from build123d import *

# Parameters (mm, degrees)
SKETCH1_R           = 2.075
SKETCH1_R_2         = 5
BOSS_EXTRUDE1_DEPTH = 5
BOSS_EXTRUDE2_DEPTH = 10


with BuildPart() as part:
    # Sketch1 → Boss-Extrude1 (new body)
    with BuildSketch(Plane(origin=(0, 0, 0), x_dir=(1, 0, 0), z_dir=(0, 1, 0))):
        with BuildLine():
            ThreePointArc((23, 37.81190645), (-17.889435034, 76.754473357), (16.937219731, 121.201897721))
            Line((16.937219731, 121.201897721), (16.937219731, 130.106631122))
            ThreePointArc((16.937219731, 130.106631122), (-26.790527996, 80.780951543), (15, 29.80360013))
            Line((15, 29.80360013), (15, 17.435595774))
            ThreePointArc((15, 17.435595774), (-20.90454496, -9.591663047), (23, 0))
            Line((23, 0), (23, 37.81190645))
        make_face()
        with Locations(Location((8, 8, 0), (0, 0, 270))):
            Circle(SKETCH1_R, mode=Mode.SUBTRACT)
        with Locations(Location((0, 0, 0), (0, 0, 270))):
            Circle(SKETCH1_R_2, mode=Mode.SUBTRACT)
        with Locations(Location((-8, -8, 0), (0, 0, 270))):
            Circle(SKETCH1_R, mode=Mode.SUBTRACT)
        with Locations(Location((-8, 8, 0), (0, 0, 270))):
            Circle(SKETCH1_R, mode=Mode.SUBTRACT)
        with Locations(Location((8, -8, 0), (0, 0, 270))):
            Circle(SKETCH1_R, mode=Mode.SUBTRACT)
    extrude(amount=BOSS_EXTRUDE1_DEPTH)

    # Sketch1_3 → Boss-Extrude2 (add)
    with BuildSketch(Plane(origin=(0, 0, 0), x_dir=(1, 0, 0), z_dir=(0, 1, 0))):
        with BuildLine():
            Line((23, 23), (23, 29))
            Line((23, 29), (23, 29.009843473))
            Line((23, 29.009843473), (23, 37.81190645))
            ThreePointArc((23, 37.81190645), (19.957969223, 37.994952611), (16.937219731, 38.398102279))
            ThreePointArc((16.937219731, 38.398102279), (-18, 79.8), (16.937219731, 121.201897721))
            Line((16.937219731, 121.201897721), (16.937219731, 130.106631122))
            ThreePointArc((16.937219731, 130.106631122), (-26.790527996, 80.780951543), (15, 29.80360013))
            Line((15, 29.80360013), (15, 23))
            Line((15, 23), (15, 17.435595774))
            Line((15, 17.435595774), (15, 0))
            ThreePointArc((15, 0), (10.606601718, -10.606601718), (0, -15))
            Line((0, -15), (0, -23))
            ThreePointArc((0, -23), (16.263455967, -16.263455967), (23, 0))
            Line((23, 0), (23, 23))
        make_face()
    extrude(amount=BOSS_EXTRUDE2_DEPTH)


solid = part.part
CAD build for the part. Positions are in the model's coordinates, mm. A direction names the side the tool comes from. Give positions to 0.01 mm unless a question says otherwise; leave off trailing zeros. Loops run counter-clockwise (first coordinate to the right, second up) from the corner with the lowest first, then second, coordinate; pieces in that order, holes last. Notation, with made-up numbers: M 82.25,54 L 133.25,54 A27 ccw 133.25,84 Z; hole C -23,89 d8. An arc over 180 degrees is marked long. One line per question, with ' | ' between items. Start each with the question number.
1. 3-axis set-ups, long thin cutter, end or side, ignore diameter. For faces 5 (the face through (-26.76, 4.93, -81.78)), 6 (the face through (-4, 5, -5)): which of +Z, -Z, +X, -X, +Y, -Y reach the whole face in a straight line?
2. Saw through at B-B on y = 8.25. Give the cut face in (x, z), plus the area to 3 significant figures.
3. Saw through at A-A on x = -13. Give the cut face in (y, z), plus the area to 3 significant figures.
4. Flat gauge pins, fed straight in: pin 1 (5 mm diameter, centred on y = 6, z = -9.5, fed in from -X); pin 2 (4 mm diameter, centred on x = 13, y = 8, fed in from +Z); pin 3 (2 mm diameter, centred on x = 17, y = 1, fed in from +Z). Where does each tip first touch, or does it go through?
5. Saw through at D-D on z = -8. Give the cut face in (x, y) (3 decimals).
6. Saw through at C-C on z = 8. Give the cut face in (x, y) (3 decimals).
7. Two-plate mould, pull along X, no slides. Class faces 1 (the face through (16.937, 5, -126)), 2 (the face through (0, 7, 19)), 3 (the face through (5.974, 2.465, 7.55)), 4 (the face through (15, 6, -18)): pulls with the +X half, pulls with the -X half, needs draft (parallel to the pull), parting line crosses it, or undercut.
8. Probe L1, parallel to X at y = 2.9, z = -8 (3 decimals); L2, parallel to X at y = 2.55, z = 8 (3 decimals); L3, parallel to Z at x = -1, y = 3.5. List the from-to ranges inside material, lowest first. Write a range as from..to.
Result sheet:
1) face 5: -X, +Y, -Y | face 6: -X, +Y
2) outline: M 0,15 A15 cw 15,0 L 15,-29.8 A50.8 ccw 16.94,-130.11 L 16.94,-121.2 A42 cw 23,-37.81 L 23,0 A23 ccw 0,23 Z | area: 1,680 mm^2
3) outline: M 0,-114.61 L 10,-114.61 L 10,-99.67 L 0,-99.67 Z; M 0,-59.93 L 10,-59.93 L 10,-44.99 L 0,-44.99 Z; M 0,-18.97 L 5,-18.97 L 5,18.97 L 0,18.97 Z | area: 488 mm^2
4) pin 1: stops at x = -21.84 | pin 2: stops at z = 20.2 | pin 3: stops at z = 16.52
5) outline: M -21.564,0 L -10.075,0 L -10.075,5 L -21.564,5 Z; M -5.925,0 L 5.925,0 L 5.925,5 L -5.925,5 Z; M 10.075,0 L 23,0 L 23,10 L 15,10 L 15,5 L 10.075,5 Z
6) outline: M -21.564,0 L -10.075,0 L -10.075,5 L -21.564,5 Z; M -5.925,0 L 5.925,0 L 5.925,5 L -5.925,5 Z; M 10.075,0 L 21.564,0 L 21.564,10 L 12.689,10 L 12.689,5 L 10.075,5 Z
7) face 1: pulls with the +X half | face 2: pulls with the -X half | face 3: undercut | face 4: undercut
8) L1: x = -21.564..-10.075, -5.925..5.925, 10.075..23 | L2: x = -21.564..-10.075, -5.925..5.925, 10.075..21.564 | L3: z = -124.02..-113.55, -46.05..-35.58, -22.98..-4.9, 4.9..22.98
